For this review, use the dimensioned drawing (mm, ordinates from the lowest corner) and the shaded views. Give positions to 0.01 mm unless a question says otherwise; leave off trailing zeros. Write each loop counter-clockwise with the first axis right and the second up, starting at its lowest first coordinate (ties: lowest second). Pieces come first, ordered by that corner, then holes. Notation, with made-up numbers: M -30.5,-25 L 5.5,-25 A22 cw 5.5,-14 Z; hole C 70,-6.5 d9. An arc over 180 degrees is marked long. One line per item, written item: value. Start each with the question number.
Item 1: Consider section A-A, the plane x = 6. Write out the cut boundary in (y, z).
Item 2: Clearance check with flat-ended pins moving along their axes: pin 1 Ø1 at (x, z) = (3.5, 1) entering from +Y; pin 2 Ø2 at (x, z) = (2.5, 2) entering from -Y; pin 3 Ø1.5 at (x, y) = (6, 10) entering from -Z. State where each tip first meets the part, or that it passes through.
Item 3: Mouldability with a two-part tool opening along Y and no side actions: class the marked faces 1, 2 and 3 as released by +Y, released by -Y, zero draft, split by the parting line, or undercut.
Item 4: To check wall thickness, follow probe 1 along Y at (x, z) = (6, 1.7); probe 2 along Y at (x, z) = (5.25, 3); probe 3 along Y at (x, z) = (3, 3). State the ranges of each line that lie inside material, in increasing order.
Item 5: Consider section C-C, the plane z = 0.85. Write out the cut boundary in (x, y).
Item 6: Consider section D-D, the plane x = 2. Write out the cut boundary in (y, z).
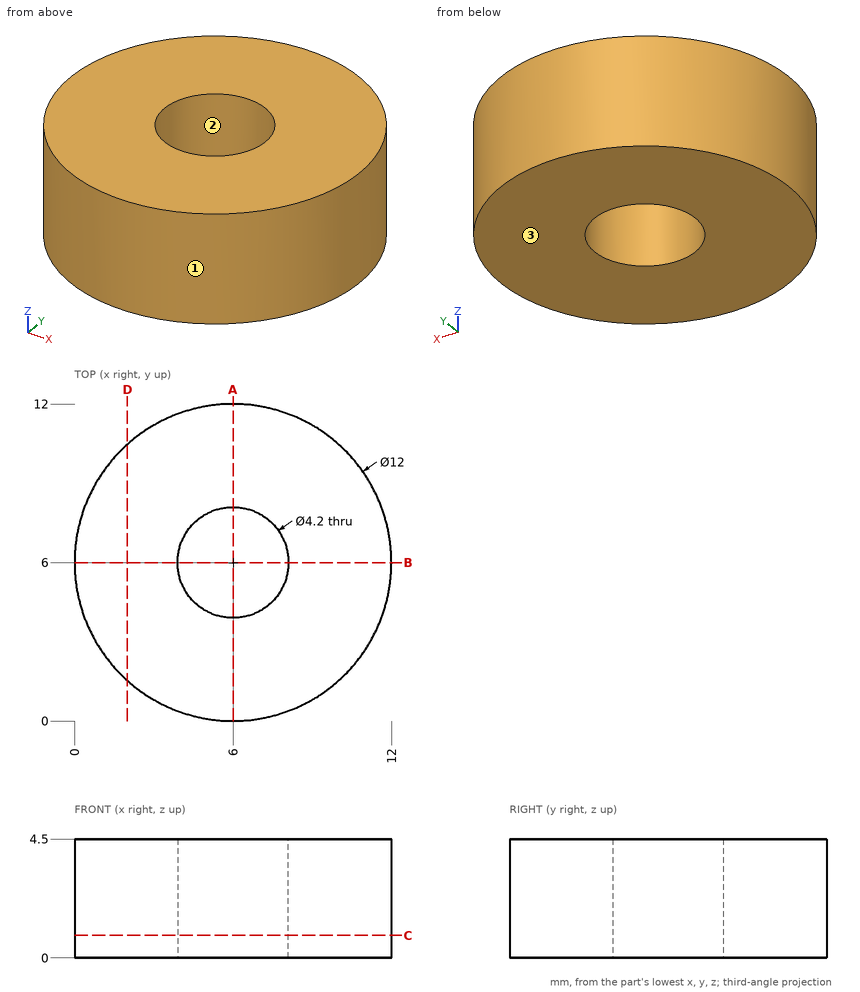
Model answer:
1. outline: M 0,0 L 3.9,0 L 3.9,4.5 L 0,4.5 Z; M 8.1,0 L 12,0 L 12,4.5 L 8.1,4.5 Z
2. pin 1: stops at y = 11.66
2. pin 2: stops at y = 0.55
2. pin 3: stops at z = 0
3. face 1: split by the parting line
3. face 2: undercut
3. face 3: zero draft
4. probe 1: y = 0 to 3.9, 8.1 to 12
4. probe 2: y = 0.05 to 4.04, 7.96 to 11.95
4. probe 3: y = 0.8 to 11.2
5. outline: C 6,6 d12; hole C 6,6 d4.2
6. outline: M 1.53,0 L 10.47,0 L 10.47,4.5 L 1.53,4.5 Z
